Input: part model. Units: mm. Frame: model coordinates. A direction names the side the tool comes from. Round coordinates to 2 decimals unless told otherwise and drop trailing zeros. Order: outer loops, then holes, each group sorted by start corner. A loop starts at its lowest first (then second) coordinate and runs counter-clockwise, first axis right, second up. Notation, with made-up numbers: (39, 47.25) -> (58, 47.25) arc R20 cw to (58, 82.25) -> close; hole circle Ø5 at (-31.5, 4). An arc over 180 degrees is marked (long way). Use a Markdown table: item, result.
from build123d import *

# Parameters (mm, degrees)
SKETCH1_W           = 20
SKETCH1_H           = 20
SKETCH1_W_2         = 56
BOSS_EXTRUDE1_DEPTH = 20
BOSS_EXTRUDE2_START = 1.55
SKETCH1_3_W         = 20
SKETCH1_3_H         = 16.9
SKETCH1_3_W_2       = 18.378378378
BOSS_EXTRUDE2_DEPTH = 16.9
SKETCH2_W           = 16.9
SKETCH2_H           = 16.9
BOSS_EXTRUDE3_DEPTH = 20
FILLET2_R           = 1


with BuildPart() as part:
    # Sketch1 → Boss-Extrude1 (new body)
    with BuildSketch(Plane(origin=(0, 0, 0), x_dir=(1, 0, 0), z_dir=(0, 1, 0))):
        with Locations((-38, 0)):
            Rectangle(SKETCH1_W, SKETCH1_H)
        Rectangle(SKETCH1_W_2, SKETCH1_H)
        with Locations((38, 0)):
            Rectangle(SKETCH1_W, SKETCH1_H)
    extrude(amount=BOSS_EXTRUDE1_DEPTH)

    # Sketch1_3 → Boss-Extrude2 (add)
    with BuildSketch(Plane(origin=(0, 0, 0), x_dir=(1, 0, 0), z_dir=(0, 1, 0)).offset(BOSS_EXTRUDE2_START)):
        with Locations((-58, 0)):
            Rectangle(SKETCH1_3_W, SKETCH1_3_H)
        with Locations((57.189189189, 0)):
            Rectangle(SKETCH1_3_W_2, SKETCH1_3_H)
    extrude(amount=BOSS_EXTRUDE2_DEPTH)

    # Sketch2 → Boss-Extrude3 (add)
    with BuildSketch(Plane(origin=(0, 20, 0), x_dir=(1, 0, 0), z_dir=(0, 1, 0))):
        with Locations((38, 0)):
            Rectangle(SKETCH2_W, SKETCH2_H)
        with Locations((-38, 0)):
            Rectangle(SKETCH2_W, SKETCH2_H)
    extrude(amount=BOSS_EXTRUDE3_DEPTH)

    # Fillet2
    fillet2_edges = [part.edges().sort_by_distance(p)[0] for p in [
        (0, 20, 10),
        (-68, 18.45, 0),
        (-68, 10, -8.45),
        (-58, 18.45, 8.45),
        (-68, 10, 8.45),
        (-58, 1.55, -8.45),
        (-58, 18.45, -8.45),
        (-68, 1.55, 0),
        (-58, 1.55, 8.45),
        (0, 20, -10),
        (57.189189189, 1.55, 8.45),
        (66.378378378, 1.55, 0),
        (66.378378378, 10, 8.45),
        (57.189189189, 18.45, -8.45),
        (66.378378378, 10, -8.45),
        (57.189189189, 18.45, 8.45),
        (66.378378378, 18.45, 0),
        (57.189189189, 1.55, -8.45),
        (46.45, 30, 8.45),
        (46.45, 30, -8.45),
        (29.55, 30, -8.45),
        (29.55, 30, 8.45),
        (46.45, 40, 0),
        (38, 40, -8.45),
        (29.55, 40, 0),
        (38, 40, 8.45),
        (-46.45, 30, -8.45),
        (-46.45, 30, 8.45),
        (-29.55, 30, 8.45),
        (-29.55, 30, -8.45),
        (-46.45, 40, 0),
        (-38, 40, 8.45),
        (-29.55, 40, 0),
        (-38, 40, -8.45),
        (0, 0, -10),
        (0, 0, 10),
    ]]
    fillet(fillet2_edges, radius=FILLET2_R)


solid = part.part
1) Contact query for flat-ended pins moving along their axis: P1, Ø4.5, axis at y = 30.5, z = -2.5, coming from the -X side; P2, Ø12, axis at x = 41, y = 32.5, coming from the +Z side; P3, Ø12, axis at y = 31.5, z = 1, coming from the +X side. Output: stop coordinate, or through.
Answer key:
| item | result |
|---|---|
| P1 | stops at x = -46.45 |
| P2 | stops at z = 8.45 |
| P3 | stops at x = 46.45 |
2) Draft query along X for faces 1 (the face through (-48, 19, 0)), 2 (the face through (29.55, 29, 0)), 3 (the face through (-1, 0, 0)). Return one class per face: released by +X, released by -X, zero draft, split by the parting line, or undercut.
Answer key:
| item | result |
|---|---|
| face 1 | released by -X |
| face 2 | undercut |
| face 3 | zero draft |
3) Cut plane C-C on z = 0.25. Return loops of the section in (x, y), and give its area (3 significant figures).
Answer key:
| item | result |
|---|---|
| outline | (-68, 2.55) arc R1 ccw to (-67, 1.55) -> (-48, 1.55) -> (-48, 0) -> (48, 0) -> (48, 1.55) -> (65.38, 1.55) arc R1 ccw to (66.38, 2.55) -> (66.38, 17.45) arc R1 ccw to (65.38, 18.45) -> (48, 18.45) -> (48, 20) -> (46.45, 20) -> (46.45, 39) arc R1 ccw to (45.45, 40) -> (30.55, 40) arc R1 ccw to (29.55, 39) -> (29.55, 20) -> (-29.55, 20) -> (-29.55, 39) arc R1 ccw to (-30.55, 40) -> (-45.45, 40) arc R1 ccw to (-46.45, 39) -> (-46.45, 20) -> (-48, 20) -> (-48, 18.45) -> (-67, 18.45) arc R1 ccw to (-68, 17.45) -> close |
| area | 3,240 mm^2 |
4) Cut plane A-A on y = 26.5. Return loops of the section in (x, z).
Answer key:
| item | result |
|---|---|
| outline | (-46.45, -7.45) arc R1 ccw to (-45.45, -8.45) -> (-30.55, -8.45) arc R1 ccw to (-29.55, -7.45) -> (-29.55, 7.45) arc R1 ccw to (-30.55, 8.45) -> (-45.45, 8.45) arc R1 ccw to (-46.45, 7.45) -> close; (29.55, -7.45) arc R1 ccw to (30.55, -8.45) -> (45.45, -8.45) arc R1 ccw to (46.45, -7.45) -> (46.45, 7.45) arc R1 ccw to (45.45, 8.45) -> (30.55, 8.45) arc R1 ccw to (29.55, 7.45) -> close |
5) Cut plane D-D on y = 14.5. Return loops of the section in (x, z), and give its area (3 significant figures).
Answer key:
| item | result |
|---|---|
| outline | (-68, -7.45) arc R1 ccw to (-67, -8.45) -> (-48, -8.45) -> (-48, -10) -> (48, -10) -> (48, -8.45) -> (65.38, -8.45) arc R1 ccw to (66.38, -7.45) -> (66.38, 7.45) arc R1 ccw to (65.38, 8.45) -> (48, 8.45) -> (48, 10) -> (-48, 10) -> (-48, 8.45) -> (-67, 8.45) arc R1 ccw to (-68, 7.45) -> close |
| area | 2,570 mm^2 |
6) Set-up query: faces 4 (the face through (-58, 10, -8.45)), 5 (the face through (-58, 1.55, 0)), 6 (the face through (57, 18.45, 0)). Return all of +Z, -Z, +X, -X, +Y, -Y with unobstructed straight access to the full face (end or side cutting, diameter ignored); none if empty.
Answer key:
| item | result |
|---|---|
| face 4 | -Z, -X, +Y, -Y |
| face 5 | +Z, -Z, -X, -Y |
| face 6 | +Z, -Z, +X, +Y |
7) Ray query, probe 1 along X at (y, z) = (24, -5.5); probe 2 along Z at (x, y) = (-60, 12); probe 3 along Y at (x, z) = (-49.5, -3.25). Return the intervals inside material, ascending.
Answer key:
| item | result |
|---|---|
| probe 1 | x = -46.45 to -29.55, 29.55 to 46.45 |
| probe 2 | z = -8.45 to 8.45 |
| probe 3 | y = 1.55 to 18.45 |
8) Cut plane B-B on x = -7. Return loops of the section in (y, z).
Answer key:
| item | result |
|---|---|
| outline | (0, -9) arc R1 ccw to (1, -10) -> (19, -10) arc R1 ccw to (20, -9) -> (20, 9) arc R1 ccw to (19, 10) -> (1, 10) arc R1 ccw to (0, 9) -> close |
